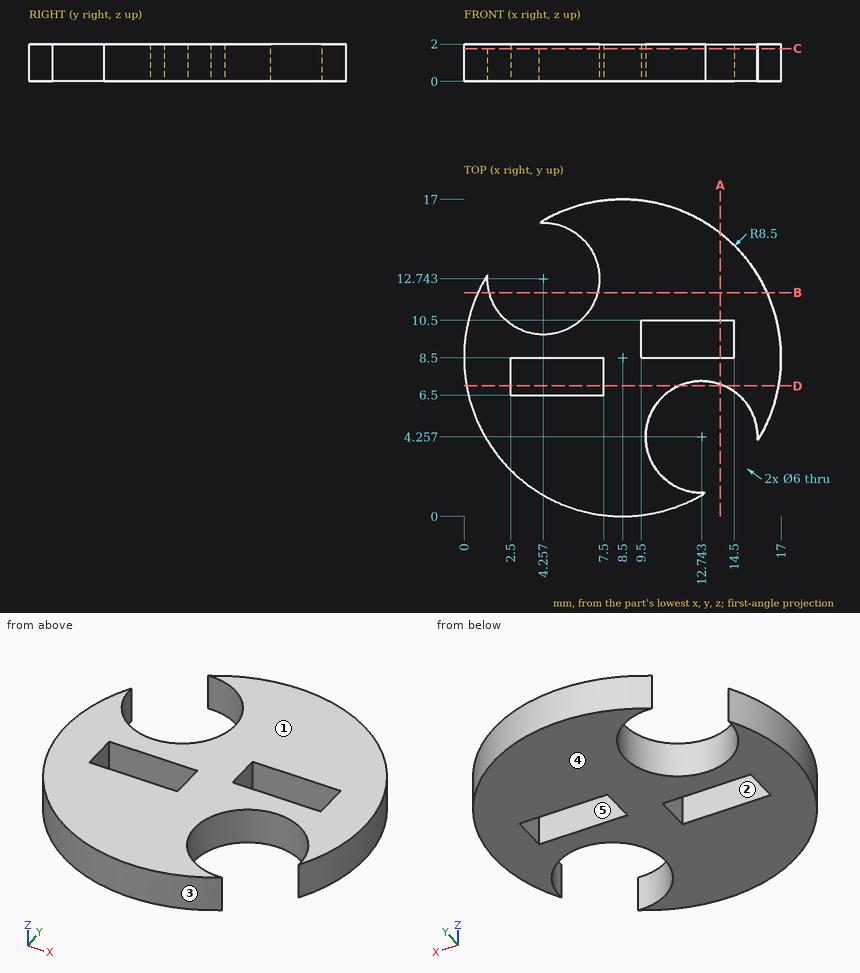
Print and shaded views of the part. All mm, measured from the part's lowest x, y and z. A direction names the side the tool comes from. Round coordinates to 2 decimals unless told otherwise and drop trailing zeros. Write each loop counter-clockwise with the first axis right and the second up, starting at its lowest first coordinate (ties: lowest second). Pieces come first, ordered by that corner, then holes. Notation, with made-up numbers: (-35, 29.25) - (-13, 29.25) arc R25 ccw to (-13, 64.25) - close; hole circle Ø3 at (82.25, 67.5). An arc over 180 degrees is marked (long way). One line per item, written item: value.
(1) Cut at D-D, the plane y = 7. Give the cut face in (x, z), plus the area to 3 significant figures.
Values follow:
outline: (0.13, 0) - (2.5, 0) - (2.5, 2) - (0.13, 2) - close; (7.5, 0) - (11.53, 0) - (11.53, 2) - (7.5, 2) - close; (13.96, 0) - (16.87, 0) - (16.87, 2) - (13.96, 2) - close
area: 18.6 mm²
(2) Cut at C-C, the plane z = 1.75. Give the cut face in (x, y) (1 decimal).
Values follow:
outline: (1.3, 13) arc R8.5 ccw to (13, 1.3) arc R3 cw (long way) to (15.7, 4) arc R8.5 ccw to (4, 15.7) arc R3 cw (long way) to start; hole (2.5, 6.5) - (7.5, 6.5) - (7.5, 8.5) - (2.5, 8.5) - close; hole (9.5, 8.5) - (14.5, 8.5) - (14.5, 10.5) - (9.5, 10.5) - close
(3) 3-axis set-ups, long thin cutter, end or side, ignore diameter. For the marked faces 1 and 2: which of +Z, -Z, +X, -X, +Y, -Y reach the whole face in a straight line?
Values follow:
face 1: +Z, +X, -X, +Y, -Y
face 2: +Z, -Z
(4) Cut at A-A, the plane x = 13.75. Give the cut face in (y, z) (1 decimal), plus the area to 3 significant figures.
Values follow:
outline: (7.1, 0) - (8.5, 0) - (8.5, 2) - (7.1, 2) - close; (10.5, 0) - (15.2, 0) - (15.2, 2) - (10.5, 2) - close
area: 12.2 mm²
(5) Wall check: probe 1 along X at (y, z) = (8.25, 1.45); probe 2 along Y at (x, z) = (10.75, 0.1) (1 decimal); probe 3 along X at (y, z) = (6.75, 0.25) (1 decimal). Give the ranges that are in metal, low to high.
Values follow:
probe 1: x = 0 to 2.5, 7.5 to 17
probe 2: y = 0.3 to 2, 6.5 to 8.5, 10.5 to 16.7
probe 3: x = 0.2 to 2.5, 7.5 to 11.1, 14.4 to 16.8
(6) Cut at B-B, the plane y = 12. Give the cut face in (x, z).
Values follow:
outline: (0.75, 0) - (1.35, 0) - (1.35, 2) - (0.75, 2) - close; (7.16, 0) - (16.25, 0) - (16.25, 2) - (7.16, 2) - close
(7) Two-plate mould, pull along X, no slides. Class the marked faces 3, 4 and 5: pulls with the +X half, pulls with the -X half, needs draft (parallel to the pull), parting line crosses it, or undercut.
Values follow:
face 3: parting line crosses it
face 4: needs draft
face 5: undercut
(8) Drop flat-ended pins along their axis: P1, Ø1, axis at y = 10, z = 1.5, coming from the -X side; P2, Ø1, axis at x = 5.5, z = 0.5, coming from the +Y side; P3, Ø0.6, axis at y = 9.5, z = 1, coming from the +X side; P4, Ø5, axis at x = 12.74, y = 4.26, coming from the -Z side. Give the stop position or say it passes through.
Values follow:
P1: stops at x = 0.06
P2: stops at y = 16.62
P3: stops at x = 16.97
P4: passes through
